from build123d import *

# Parameters (mm, degrees)
SKETCH1_R           = 10
BOSS_EXTRUDE1_DEPTH = 1


with BuildPart() as part:
    # Sketch1 → Boss-Extrude1 (new body)
    with BuildSketch(Plane(origin=(0, 0, 0), x_dir=(1, 0, 0), z_dir=(0, 1, 0))):
        with Locations(Location((0, 0, 0), (0, 0, 270))):
            Circle(SKETCH1_R)
        with BuildLine():
            Line((-0.5, 6), (0.5, 6))
            ThreePointArc((0.5, 6), (6.5, 0), (0.5, -6))
            Line((0.5, -6), (-0.5, -6))
            ThreePointArc((-0.5, -6), (-6.5, 0), (-0.5, 6))
        make_face(mode=Mode.SUBTRACT)
    extrude(amount=BOSS_EXTRUDE1_DEPTH)


solid = part.part
Can you work these out from the model? Positions are in its coordinate system, mm. A direction names the side the tool comes from. Round coordinates to 2 decimals unless told otherwise and drop trailing zeros. Loops run counter-clockwise (first coordinate to the right, second up) from the corner with the lowest first, then second, coordinate; pieces in that order, holes last. Notation, with made-up numbers: (89.5, 70) - (133.5, 70) arc R15 cw to (133.5, 79) - close; hole circle Ø9 at (81, 18.25). An arc over 180 degrees is marked (long way). Use CSV: the item, a comma, the result in double quotes. Start each with the question number.
1) Please list where these lines run through material, in increasing order: probe 1 along Z at (x, y) = (5.75, 0.8); probe 2 along Z at (x, y) = (-4.5, 0.9); probe 3 along X at (y, z) = (0.8, -3.5). Write a range as [from, to].
2) For faces 1 (the flat face through (-7, 1, 0)), 2 (the cylindrical face through (-6.5, 0.5, 0.1)), which set-ups out of +Z, -Z, +X, -X, +Y, -Y let a thin tool reach every point of the face, with its end or its side?
3) If we section it at A-A on x = 0: Write out the boundary of the cut face in (y, z).
4) We'd pull the mould along Z, two halves only. Please class faces 3 (the cylindrical face through (6.5, 0.5, -0.1)), 4 (the cylindrical face through (-9.76, 0.49, -2.17)), 5 (the flat face through (0, 0.5, 6)), 6 (the flat face through (-7, 0, 0)): released by +Z, released by -Z, zero draft, split by the parting line, or undercut.
5) If we section it at D-D on x = 7.75: Write out the boundary of the cut face in (y, z).
6) If we section it at B-B on z = 0: Write out the boundary of the cut face in (x, y).
7) If we section it at C-C on y = 0.35: Write out the boundary of the cut face in (x, z), plus the area to 3 significant figures.
Geometry results:
1,probe 1,"z = [-8.18, -2.9], [2.9, 8.18]"
1,probe 2,"z = [-8.93, -4.47], [4.47, 8.93]"
1,probe 3,"x = [-9.37, -5.37], [5.37, 9.37]"
2,face 1,"+Z, -Z, +X, -X, +Y"
2,face 2,"+Y, -Y"
3,outline,"(0, -10) - (1, -10) - (1, -6) - (0, -6) - close; (0, 6) - (1, 6) - (1, 10) - (0, 10) - close"
4,face 3,"undercut"
4,face 4,"split by the parting line"
4,face 5,"undercut"
4,face 6,"zero draft"
5,outline,"(0, -6.32) - (1, -6.32) - (1, 6.32) - (0, 6.32) - close"
6,outline,"(-10, 0) - (-6.5, 0) - (-6.5, 1) - (-10, 1) - close; (6.5, 0) - (10, 0) - (10, 1) - (6.5, 1) - close"
7,outline,"circle Ø20 at (0, 0); hole (-0.5, -6) - (0.5, -6) arc R6 ccw to (0.5, 6) - (-0.5, 6) arc R6 ccw to start"
7,area,"189 mm2"
